```python
from build123d import *

# Parameters (mm, degrees)
F0_W     = 15
F0_H     = 4
F3_SIZE  = 5
F6_D     = 6.6
F6_DEPTH = 10
F6_TIP   = 1.9828400428
F7_SIZE  = 1


with BuildPart() as f1:
    # F0 (on Front) → F1 (revolve)
    with BuildSketch(Plane.XZ):
        Polygon((-30, 8.75), (0, 8.75), (0, 12.75), (0, 23.5), (-30, 23.5), align=None)
        with Locations((7.5, 10.75)):
            Rectangle(F0_W, F0_H)
    revolve(axis=Axis((-19.2540567368, 0, 0), (-1, 0, 0)))

    # F3
    f3_edges = [f1.edges().sort_by_distance(p)[0] for p in [
        (-30, 0, -8.75),
    ]]
    chamfer(f3_edges, length=F3_SIZE)

    # F6
    with Locations(Plane(origin=(0, 0, -25), x_dir=(1, 0, 0), z_dir=(0, 0, -1))):
        with Locations((-18, 0)):
            Hole(F6_D / 2, depth=F6_DEPTH)
            with Locations((0, 0, -(F6_DEPTH + F6_TIP / 2))):  # 118° drill point
                Cone(0, F6_D / 2, F6_TIP, mode=Mode.SUBTRACT)

    # F7
    f7_edges = [f1.edges().sort_by_distance(p)[0] for p in [
        (-30, 0, -23.5),
        (0, 0, -23.5),
        (15, 0, -12.75),
        (15, 0, -8.75),
    ]]
    chamfer(f7_edges, length=F7_SIZE)


solid = f1.part
```
Geometry check sheet. Reference: the model listing, model coordinates, mm. A direction names the side the tool comes from. Round coordinates to 2 decimals unless told otherwise and drop trailing zeros. Loops run counter-clockwise (first coordinate to the right, second up) from the corner with the lowest first, then second, coordinate; pieces in that order, holes last. Notation, with made-up numbers: (8, 12.5) - (25, 12.5) arc R14 cw to (25, 31.5) - close; hole circle Ø6 at (-4.5, -13.75). An arc over 180 degrees is marked (long way). Write item = value, one per line. Start each with the question number.
1. Set-up check for faces 1 (the face through (7.098, -12.447, -2.764)), 2 (the face through (-30, -10, -10)), 3 (the face through (-14.7, -0.1, -19.2)): record each of +Z, -Z, +X, -X, +Y, -Y from which the full face is reachable in a straight line by a thin tool's end or side.
2. Thickness scan on line 1 (Y direction, x = -10, z = 0); line 2 (X direction, y = -1, z = 18.5); line 3 (Z direction, x = -17, y = -1.5). Record the ranges inside material, lowest first.
3. Mould release check, pull along X, two halves, no side actions. Record for faces 4 (the face through (-5.227, -5.324, -6.944)), 5 (the face through (0, -10, -10)), 6 (the face through (-25.31, 2.72, 8.64)), 7 (the face through (-17.47, 0.22, -13.36)): released by +X, released by -X, zero draft, split by the parting line, or undercut.
4. Section check B-B on x = -11. Enter the section's corners in (y, z).
5. Depth check by flat-ended pin: pin 1 (3 mm diameter, centred on x = 8, z = -5.5, fed in from -Y); pin 2 (3 mm diameter, centred on x = -20, y = -18, fed in from -Z); pin 3 (1.5 mm diameter, centred on x = -19.5, z = 13, fed in from +Y); pin 4 (5 mm diameter, centred on x = 9.5, y = -16, fed in from +Z). Enter the tip coordinate at first touch or a pass-through.
6. Section check C-C on x = 9.5. Enter the section's corners in (y, z), then the cut area to 3 significant figures.
7. Section check A-A on z = 0. Enter the section's corners in (x, y).
Working result:
q1.face_1 = +X
q1.face_2 = +Z, -Z, -X, +Y, -Y
q1.face_3 = -Z
q2.line_1 = -23.5 to -8.75, 8.75 to 23.5
q2.line_2 = -30 to 0
q2.line_3 = -14.1 to -8.62, 8.62 to 23.45
q3.face_4 = zero draft
q3.face_5 = released by +X
q3.face_6 = released by -X
q3.face_7 = undercut
q4.outline = circle Ø47 at (0, 0); hole circle Ø17.5 at (0, 0)
q5.pin_1 = -12.11
q5.pin_2 = -16.73
q5.pin_3 = 20.05
q5.pin_4 = through
q6.outline = circle Ø25.5 at (0, 0); hole circle Ø17.5 at (0, 0)
q6.area = 270 mm^2
q7.outline = (-30, -22.5) - (-29, -23.5) - (-1, -23.5) - (0, -22.5) - (0, -12.75) - (14, -12.75) - (15, -11.75) - (15, -9.75) - (14, -8.75) - (-25, -8.75) - (-30, -13.75) - close; (-30, 13.75) - (-25, 8.75) - (14, 8.75) - (15, 9.75) - (15, 11.75) - (14, 12.75) - (0, 12.75) - (0, 22.5) - (-1, 23.5) - (-29, 23.5) - (-30, 22.5) - close
